```python
from build123d import *

# Parameters (mm, degrees)
SKETCH1_W           = 38
SKETCH1_H           = 13
SKETCH1_R           = 2.9
SKETCH1_R_2         = 2.5
BOSS_EXTRUDE1_DEPTH = 5.6


with BuildPart() as part:
    # Sketch1 → Boss-Extrude1 (new body)
    with BuildSketch(Plane.XY):
        Rectangle(SKETCH1_W, SKETCH1_H)
        Circle(SKETCH1_R, mode=Mode.SUBTRACT)
        with Locations((-12, 0)):
            Circle(SKETCH1_R_2, mode=Mode.SUBTRACT)
        with Locations((12, 0)):
            Circle(SKETCH1_R_2, mode=Mode.SUBTRACT)
    extrude(amount=BOSS_EXTRUDE1_DEPTH)


solid = part.part
```
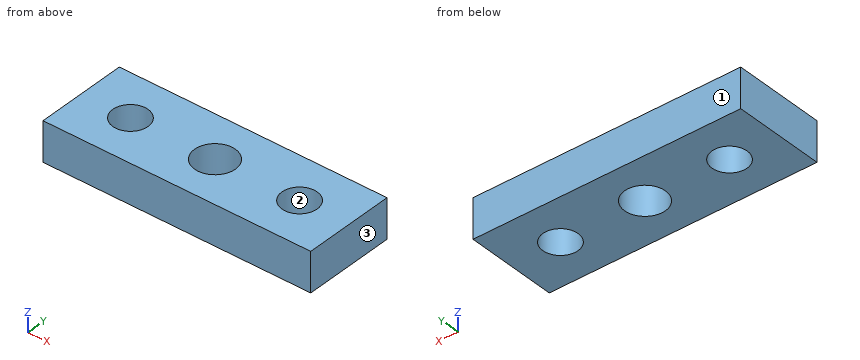
Check sheet for the modelled part. Datum: model origin and axes. Units: mm. Face numbers are marked on the shaded views. Give positions to 0.01 mm unless a question says otherwise; leave off trailing zeros. Order: outer loops, then holes, each group sorted by start corner. A loop starts at its lowest first (then second) coordinate and runs counter-clockwise, first axis right, second up. Notation, with made-up numbers: (18.5, -18.5) -> (75.5, -18.5) arc R18 ccw to (75.5, 16.5) -> close; hole circle Ø6 at (51.5, 45.25). An arc over 180 degrees is marked (long way). Use CSV: the item, a comma, the result in double quotes. Start each with the question number.
1) Sectioned sample at C-C, the plane y = 0. Record the boundary of the cut face in (x, z).
2) Sectioned sample at A-A, the plane x = 12. Record the boundary of the cut face in (y, z), plus the area to 3 significant figures.
3) Go/stop test with a flat-tipped pin: P1, Ø4.5, axis at x = -12, y = 0, coming from the +Z side. Record where the tip stops, or that it passes through.
4) Sectioned sample at D-D, the plane x = 0. Record the boundary of the cut face in (y, z), plus the area to 3 significant figures.
5) Material ranges on line 1 (Y direction, x = 0, z = 1.9); line 2 (X direction, y = -1.75, z = 1.3); line 3 (Y direction, x = 12, z = 3.2), recorded low to high. Write a range as from..to.
6) Sectioned sample at B-B, the plane z = 1.2. Record the boundary of the cut face in (x, y), plus the area to 3 significant figures.
7) Mould release check, pull along X, two halves, no side actions. Record for the marked faces 1, 2 and 3: released by +X, released by -X, zero draft, split by the parting line, or undercut.
Recorded:
1,outline,"(-19, 0) -> (-14.5, 0) -> (-14.5, 5.6) -> (-19, 5.6) -> close; (-9.5, 0) -> (-2.9, 0) -> (-2.9, 5.6) -> (-9.5, 5.6) -> close; (2.9, 0) -> (9.5, 0) -> (9.5, 5.6) -> (2.9, 5.6) -> close; (14.5, 0) -> (19, 0) -> (19, 5.6) -> (14.5, 5.6) -> close"
2,outline,"(-6.5, 0) -> (-2.5, 0) -> (-2.5, 5.6) -> (-6.5, 5.6) -> close; (2.5, 0) -> (6.5, 0) -> (6.5, 5.6) -> (2.5, 5.6) -> close"
2,area,"44.8 mm2"
3,P1,"through"
4,outline,"(-6.5, 0) -> (-2.9, 0) -> (-2.9, 5.6) -> (-6.5, 5.6) -> close; (2.9, 0) -> (6.5, 0) -> (6.5, 5.6) -> (2.9, 5.6) -> close"
4,area,"40.3 mm2"
5,line 1,"-6.5..-2.9, 2.9..6.5"
5,line 2,"-19..-13.79, -10.21..-2.31, 2.31..10.21, 13.79..19"
5,line 3,"-6.5..-2.5, 2.5..6.5"
6,outline,"(-19, -6.5) -> (19, -6.5) -> (19, 6.5) -> (-19, 6.5) -> close; hole circle Ø5 at (-12, 0); hole circle Ø5.8 at (0, 0); hole circle Ø5 at (12, 0)"
6,area,"428 mm2"
7,face 1,"zero draft"
7,face 2,"undercut"
7,face 3,"released by +X"
